CAD build for the part. Positions are in the model's coordinates, mm. Face numbers are marked on the shaded views. Coordinates: 2 decimals unless noted, no trailing zeros. Write each loop counter-clockwise with the first axis right and the second up, starting at its lowest first coordinate (ties: lowest second). Pieces come first, ordered by that corner, then holes. Notation, with made-up numbers: M -30.5,49 L 11.5,49 A10 ccw 11.5,67 Z; hole C -25.75,10 d10. An arc over 180 degrees is marked long. Answer as CSV lines item,"result". Start each with the question number.
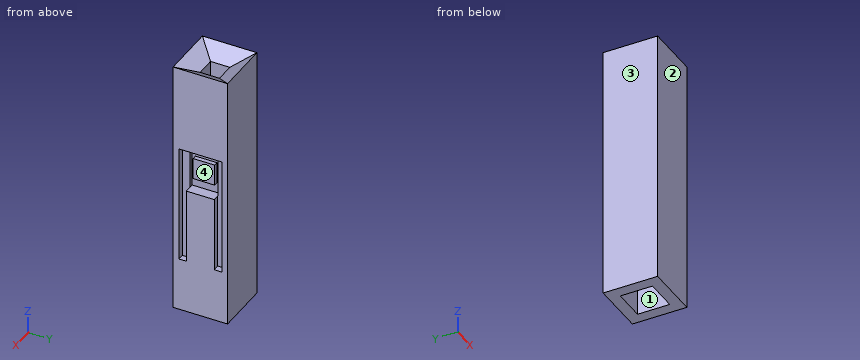
Autodesk Fusion 360 part; units mm, degrees
sketch "Sketch1" plane through (0, 0, 0) normal (0, 0, 1) x (1, 0, 0)
  line L0 (1.27, -1.27) -> (-1.27, -1.27)
  line L1 (-1.27, -1.27) -> (-1.27, 1.27)
  line L2 (-1.27, 1.27) -> (1.27, 1.27)
  line L3 (1.27, 1.27) -> (1.27, -1.27)
  line L4 (1.27, -1.27) -> (-1.27, 1.27) construction
  line L5 (-1.27, -1.27) -> (1.27, 1.27) construction
  dimension "d1" = 2.54
  dimension "d2" = 2.54
extrude "Extrude1" add sketch "Sketch1" along normal blind 12
sketch "Sketch2" plane through (0, 0, 12) normal (0, 0, 1) x (-1, 0, 0)
  line L0 (-1.27, -1.27) -> (1.27, -1.27)
  line L1 (1.27, -1.27) -> (1.27, 1.27)
  line L2 (1.27, 1.27) -> (-1.27, 1.27)
  line L3 (-1.27, 1.27) -> (-1.27, -1.27)
  line L4 (-0.45, 0.45) -> (0.45, 0.45)
  line L5 (0.45, 0.45) -> (0.45, -0.45)
  line L6 (0.45, -0.45) -> (-0.45, -0.45)
  line L7 (-0.45, -0.45) -> (-0.45, 0.45)
  line L8 (-0.45, 0.45) -> (0.45, -0.45) construction
  line L9 (0.45, 0.45) -> (-0.45, -0.45) construction
  dimension "d5" = 0.9
  dimension "d6" = 0.9
extrude "Extrude2" cut sketch "Sketch2" against normal blind 0.5 contours L4 L5 L6 L7
loft "Loft1" cut profiles "Sketch2" section 1 section 2 face at (0.15, -0.15, 11.5)
extrude "Extrude3" cut 1 faces at (0.15, -0.15, 11.5) along direction (0, 0, -1) blind 8
sketch "Sketch3" plane through (1.27, 0, 0) normal (1, 0, 0) x (0, 1, 0)
  line L0 (-1.27, 0) -> (1.27, 0)
  line L1 (1.27, 0) -> (1.27, 12)
  line L2 (1.27, 12) -> (-1.27, 12)
  line L3 (-1.27, 12) -> (-1.27, 0)
  line L4 (1, 8) -> (-1, 8)
  line L5 (-1, 8) -> (-1, 2.5)
  line L6 (-1, 2.5) -> (1, 2.5)
  line L7 (1, 2.5) -> (1, 8)
  line L8 (1, 8) -> (-1, 2.5) construction
  line L9 (-1, 8) -> (1, 2.5) construction
  line L10 (0.6487, 2.5073) -> (-0.6513, 2.5073)
  line L11 (-0.6513, 2.5073) -> (-0.6513, 6.0073)
  line L12 (-0.6513, 6.0073) -> (0.6487, 6.0073)
  line L13 (0.6487, 6.0073) -> (0.6487, 2.5073)
  line L14 (0.6487, 2.5073) -> (-0.6513, 6.0073) construction
  line L15 (-0.6513, 2.5073) -> (0.6487, 6.0073) construction
  line L16 (-0.6513, 6.0073) -> (0.6554, 6.0073)
  line L17 (0.6554, 6.0073) -> (0.6554, 8.0073)
  line L18 (0.6554, 8.0073) -> (-0.6513, 8.0073)
  line L19 (-0.6513, 8.0073) -> (-0.6513, 6.0073)
  line L20 (0.5, 6.5) -> (-0.5, 6.5)
  line L21 (-0.5, 6.5) -> (-0.5, 7.5)
  line L22 (-0.5, 7.5) -> (0.5, 7.5)
  line L23 (0.5, 7.5) -> (0.5, 6.5)
  line L24 (0.5, 6.5) -> (-0.5, 7.5) construction
  line L25 (-0.5, 6.5) -> (0.5, 7.5) construction
  line L26 (-1.27, 6) -> (-0.6513, 6.0073)
  line L27 (0.6554, 6.0073) -> (1.27, 6)
  line L28 (0.6487, 2.5073) -> (1, 2.5)
  line L29 (-0.6513, 2.5073) -> (-1, 2.5)
  point P0 (0, 5.25)
  point P1 (-0.0013, 4.2573)
  point P2 (0, 7)
  dimension "d11" = 5.5
  dimension "d12" = 2.5
  dimension "d13" = 1.3
  dimension "d14" = 3.5
  dimension "d15" = 2
  dimension "d16" = 1
  dimension "d17" = 1
extrude "Extrude4" cut sketch "Sketch3" against normal blind 0.3 contours L5 L11 L26 L29 | L4 L5 L19 L26 | L4 L7 L17 L27 | L7 L13 L16 L27 L28
extrude "Extrude5" cut sketch "Sketch3" against normal blind 0.5 contours L4 L12 L16 L17 L19
extrude "Extrude6" cut sketch "Sketch3" against normal blind 0.3 contours L20 L21 L22 L23
sketch "Sketch4" plane through (0, 0, 0) normal (0, 0, -1) x (1, 0, 0)
  line L0 (-1.27, -1.27) -> (1.27, -1.27)
  line L1 (1.27, -1.27) -> (1.27, 1.27)
  line L2 (1.27, 1.27) -> (-1.27, 1.27)
  line L3 (-1.27, 1.27) -> (-1.27, -1.27)
  line L4 (0.75, -0.75) -> (-0.75, -0.75)
  line L5 (-0.75, -0.75) -> (-0.75, 0.75)
  line L6 (-0.75, 0.75) -> (0.75, 0.75)
  line L7 (0.75, 0.75) -> (0.75, -0.75)
  line L8 (0.75, -0.75) -> (-0.75, 0.75) construction
  line L9 (-0.75, -0.75) -> (0.75, 0.75) construction
  dimension "d24" = 1.5
  dimension "d25" = 1.5
extrude "Extrude7" cut sketch "Sketch4" against normal blind 2 contours L4 L5 L6 L7
sketch "Sketch5" plane through (0, 0, 2) normal (0, 0, -1) x (1, 0, 0)
  line L0 (0.75, 0.75) -> (-0.75, 0.75)
  line L1 (-0.75, 0.75) -> (-0.75, -0.75)
  line L2 (-0.75, -0.75) -> (0.75, -0.75)
  line L3 (0.75, -0.75) -> (0.75, 0.75)
  circle A0 centre (0, 0) radius 0.725
  dimension "d28" = 1.45
extrude "Extrude8" add sketch "Sketch5" along normal blind 0.1 contours A0
1) Two-plate mould, pull along X, no slides. Class the marked faces 1, 2, 3 and 4: pulls with the +X half, pulls with the -X half, needs draft (parallel to the pull), parting line crosses it, or undercut.
2) Probe L1, parallel to Y at x = 0.1, z = 6.5; L2, parallel to X at y = 0, z = 0.75. List the from-to ranges inside material, lowest first. Write a range as [from, to].
3) Band-saw the part on A-A, the plane z = 9.25. List the corners of the cut face in (x, y).
4) Band-saw the part on B-B, the plane z = 5.25. List the corners of the cut face in (x, y), plus the area to 3 significant figures.
Result sheet:
1,face 1,"undercut"
1,face 2,"needs draft"
1,face 3,"pulls with the -X half"
1,face 4,"pulls with the +X half"
2,L1,"y = [-1.27, -0.45], [0.45, 1.27]"
2,L2,"x = [-1.27, -0.75], [0.75, 1.27]"
3,outline,"M -1.27,-1.27 L 1.27,-1.27 L 1.27,1.27 L -1.27,1.27 Z; hole M -0.45,-0.45 L 0.45,-0.45 L 0.45,0.45 L -0.45,0.45 Z"
4,outline,"M -1.27,-1.27 L 1.27,-1.27 L 1.27,-1 L 0.97,-1 L 0.97,-0.65 L 1.27,-0.65 L 1.27,0.65 L 0.97,0.65 L 0.97,1 L 1.27,1 L 1.27,1.27 L -1.27,1.27 Z; hole M -0.45,-0.45 L 0.45,-0.45 L 0.45,0.45 L -0.45,0.45 Z"
4,area,"5.43 mm²"
